```python
from build123d import *

# Parameters (mm, degrees)
F0_W     = 80
F0_H     = 80
F1_DEPTH = 3
F3_DEPTH = 25
F4_R     = 3.75
F5_DEPTH = 25


with BuildPart() as f1:
    # F0 (on Top) → F1 (new body)
    with BuildSketch(Plane.XY):
        Rectangle(F0_W, F0_H)
    extrude(amount=F1_DEPTH)

    # F2 (on face) → F3 (cut)
    with BuildSketch(Plane.XY.offset(3)):
        with BuildLine():
            ThreePointArc((25.0727558965, 11.2963229308), (23.3008846492, 7.5709163622), (26.9240976399, 5.5984789253))
            ThreePointArc((26.9240976399, 5.5984789253), (26.1540541981, 8.4979673453), (25.0727558965, 11.2963229308))
        make_face()
        with BuildLine():
            ThreePointArc((25.0727558965, 11.2963229308), (26.1540541981, 8.4979673453), (26.9240976399, 5.5984789253))
            ThreePointArc((26.9240976399, 5.5984789253), (28.5320922892, 6.669051044), (29.1540541981, 8.4979673453))
            ThreePointArc((29.1540541981, 8.4979673453), (27.8505366022, 10.9722242949), (25.0727558965, 11.2963229308))
        make_face()
        with BuildLine():
            ThreePointArc((29.1540541981, -8.4979673453), (28.5320922892, -6.669051044), (26.9240976399, -5.5984789253))
            ThreePointArc((26.9240976399, -5.5984789253), (26.1540541981, -8.4979673453), (25.0727558965, -11.2963229308))
            ThreePointArc((25.0727558965, -11.2963229308), (27.8505366022, -10.9722242949), (29.1540541981, -8.4979673453))
        make_face()
        with BuildLine():
            ThreePointArc((25.0727558965, -11.2963229308), (26.1540541981, -8.4979673453), (26.9240976399, -5.5984789253))
            ThreePointArc((26.9240976399, -5.5984789253), (23.3008846492, -7.5709163622), (25.0727558965, -11.2963229308))
        make_face()
        with BuildLine():
            ThreePointArc((13.6444735922, 23.8763133752), (14.4007386812, 19.8209163622), (18.4913492013, 20.3548521172))
            ThreePointArc((18.4913492013, 20.3548521172), (16.164094438, 22.2479673453), (13.6444735922, 23.8763133752))
        make_face()
        with BuildLine():
            ThreePointArc((13.6444735922, 23.8763133752), (16.164094438, 22.2479673453), (18.4913492013, 20.3548521172))
            ThreePointArc((18.4913492013, 20.3548521172), (18.990909279, 21.2434187626), (19.164094438, 22.2479673453))
            ThreePointArc((19.164094438, 22.2479673453), (17.0129576374, 25.1253674337), (13.6444735922, 23.8763133752))
        make_face()
        with BuildLine():
            ThreePointArc((19.164094438, -22.2479673453), (18.990909279, -21.2434187626), (18.4913492013, -20.3548521172))
            ThreePointArc((18.4913492013, -20.3548521172), (16.164094438, -22.2479673453), (13.6444735922, -23.8763133752))
            ThreePointArc((13.6444735922, -23.8763133752), (17.0129576374, -25.1253674337), (19.164094438, -22.2479673453))
        make_face()
        with BuildLine():
            ThreePointArc((13.6444735922, -23.8763133752), (16.164094438, -22.2479673453), (18.4913492013, -20.3548521172))
            ThreePointArc((18.4913492013, -20.3548521172), (14.4007386812, -19.8209163622), (13.6444735922, -23.8763133752))
        make_face()
        with BuildLine():
            ThreePointArc((-2.9955338657, 27.3363636364), (0, 24.5), (2.9955338657, 27.3363636364))
            ThreePointArc((2.9955338657, 27.3363636364), (0, 27.5), (-2.9955338657, 27.3363636364))
        make_face()
        with BuildLine():
            ThreePointArc((-2.9955338657, 27.3363636364), (0, 27.5), (2.9955338657, 27.3363636364))
            ThreePointArc((2.9955338657, 27.3363636364), (2.9988832586, 27.4181513503), (3, 27.5))
            ThreePointArc((3, 27.5), (-0.0818486497, 30.4988832586), (-2.9955338657, 27.3363636364))
        make_face()
        with BuildLine():
            ThreePointArc((3, -27.5), (2.9988832586, -27.4181513503), (2.9955338657, -27.3363636364))
            ThreePointArc((2.9955338657, -27.3363636364), (0, -27.5), (-2.9955338657, -27.3363636364))
            ThreePointArc((-2.9955338657, -27.3363636364), (-0.0818486497, -30.4988832586), (3, -27.5))
        make_face()
        with BuildLine():
            ThreePointArc((-2.9955338657, -27.3363636364), (0, -27.5), (2.9955338657, -27.3363636364))
            ThreePointArc((2.9955338657, -27.3363636364), (0, -24.5), (-2.9955338657, -27.3363636364))
        make_face()
        with BuildLine():
            ThreePointArc((-13.164094438, 22.2479673453), (-13.2866943496, 23.0968305447), (-13.6444735922, 23.8763133752))
            ThreePointArc((-13.6444735922, 23.8763133752), (-16.164094438, 22.2479673453), (-18.4913492013, 20.3548521172))
            ThreePointArc((-18.4913492013, 20.3548521172), (-15.1595458553, 19.4211525044), (-13.164094438, 22.2479673453))
        make_face()
        with BuildLine():
            ThreePointArc((-18.4913492013, 20.3548521172), (-16.164094438, 22.2479673453), (-13.6444735922, 23.8763133752))
            ThreePointArc((-13.6444735922, 23.8763133752), (-17.9274501949, 24.6750183284), (-18.4913492013, 20.3548521172))
        make_face()
        with BuildLine():
            ThreePointArc((-18.4913492013, -20.3548521172), (-17.9274501949, -24.6750183284), (-13.6444735922, -23.8763133752))
            ThreePointArc((-13.6444735922, -23.8763133752), (-16.164094438, -22.2479673453), (-18.4913492013, -20.3548521172))
        make_face()
        with BuildLine():
            ThreePointArc((-18.4913492013, -20.3548521172), (-16.164094438, -22.2479673453), (-13.6444735922, -23.8763133752))
            ThreePointArc((-13.6444735922, -23.8763133752), (-13.2866943496, -23.0968305447), (-13.164094438, -22.2479673453))
            ThreePointArc((-13.164094438, -22.2479673453), (-15.1595458553, -19.4211525044), (-18.4913492013, -20.3548521172))
        make_face()
        with BuildLine():
            ThreePointArc((-23.1540541981, 8.4979673453), (-23.6797972485, 10.1944497494), (-25.0727558965, 11.2963229308))
            ThreePointArc((-25.0727558965, 11.2963229308), (-26.1540541981, 8.4979673453), (-26.9240976399, 5.5984789253))
            ThreePointArc((-26.9240976399, 5.5984789253), (-24.3251378968, 6.1199292542), (-23.1540541981, 8.4979673453))
        make_face()
        with BuildLine():
            ThreePointArc((-26.9240976399, 5.5984789253), (-26.1540541981, 8.4979673453), (-25.0727558965, 11.2963229308))
            ThreePointArc((-25.0727558965, 11.2963229308), (-29.007223747, 9.4250183284), (-26.9240976399, 5.5984789253))
        make_face()
        with BuildLine():
            ThreePointArc((-26.9240976399, -5.5984789253), (-29.007223747, -9.4250183284), (-25.0727558965, -11.2963229308))
            ThreePointArc((-25.0727558965, -11.2963229308), (-26.1540541981, -8.4979673453), (-26.9240976399, -5.5984789253))
        make_face()
        with BuildLine():
            ThreePointArc((-26.9240976399, -5.5984789253), (-26.1540541981, -8.4979673453), (-25.0727558965, -11.2963229308))
            ThreePointArc((-25.0727558965, -11.2963229308), (-23.6797972485, -10.1944497494), (-23.1540541981, -8.4979673453))
            ThreePointArc((-23.1540541981, -8.4979673453), (-24.3251378968, -6.1199292542), (-26.9240976399, -5.5984789253))
        make_face()
    extrude(amount=-F3_DEPTH, mode=Mode.SUBTRACT)

    # F4 (on face) → F5 (cut)
    with BuildSketch(Plane.XY.offset(3)):
        with Locations((-33.1107974052, 32.4715934694)):
            Circle(F4_R)
    extrude(amount=-F5_DEPTH, mode=Mode.SUBTRACT)


solid = f1.part
```
Model file for the job. Use its own axes, mm. Give positions to 0.01 mm unless a question says otherwise; leave off trailing zeros. Order: outer loops, then holes, each group sorted by start corner. A loop starts at its lowest first (then second) coordinate and runs counter-clockwise, first axis right, second up.
1) Saw through at C-C, the plane x = -33.5. Write the cut outline in (y, z), then the cut area to 3 significant figures.
2) Saw through at D-D, the plane x = 15. Write the cut outline in (y, z), then the cut area to 3 significant figures.
3) Saw through at B-B, the plane y = -29.5. Write the cut outline in (x, z).
4) Mould opens along X. For faces 1 (the cylindrical face through (-36.857, 32.636, 1.521)), 2 (the flat face through (-40, -1, 1)), 3 (the flat face through (-1, 40, 1)) say: +X half, -X half, draft (parallel to the pull), parting line (faces both ways), or undercut.
5) Saw through at A-A, the plane x = 0. Write the cut outline in (y, z).
6) Wall check: probe 1 along Y at (x, z) = (25, 0.7); probe 2 along Y at (x, z) = (-1, 2.25); probe 3 along X at (y, z) = (-8, 0.4). Give the ranges that are in metal, low to high.
Computed:
1. outline: (-40, 0) - (28.74, 0) - (28.74, 3) - (-40, 3) - close; (36.2, 0) - (40, 0) - (40, 3) - (36.2, 3) - close
1. area: 218 mm2
2. outline: (-40, 0) - (-25.01, 0) - (-25.01, 3) - (-40, 3) - close; (-19.48, 0) - (19.48, 0) - (19.48, 3) - (-19.48, 3) - close; (25.01, 0) - (40, 0) - (40, 3) - (25.01, 3) - close
2. area: 207 mm2
3. outline: (-40, 0) - (-2.24, 0) - (-2.24, 3) - (-40, 3) - close; (2.24, 0) - (40, 0) - (40, 3) - (2.24, 3) - close
4. face 1: undercut
4. face 2: -X half
4. face 3: draft
5. outline: (-40, 0) - (-30.5, 0) - (-30.5, 3) - (-40, 3) - close; (-24.5, 0) - (24.5, 0) - (24.5, 3) - (-24.5, 3) - close; (30.5, 0) - (40, 0) - (40, 3) - (30.5, 3) - close
6. probe 1: y = -40 to -11.27, -5.73 to 5.73, 11.27 to 40
6. probe 2: y = -40 to -30.33, -24.67 to 24.67, 30.33 to 40
6. probe 3: x = -40 to -29.11, -23.2 to 23.2, 29.11 to 40
